Could you check a few things on this model? Use its own coordinates, in mm. A direction names the side the tool comes from. Coordinates: 2 decimals unless noted, no trailing zeros. Loops run counter-clockwise (first coordinate to the right, second up) from the corner with the lowest first, then second, coordinate; pieces in that order, holes last. Notation, with made-up numbers: M 54,-20 L 83,-20 A33 cw 83,10 Z; hole C 84,-3.75 d1. An arc over 180 degrees is marked long. Use one line per item in the form item = value. Start each with the question number.
Autodesk Inventor part; units mm, degrees
ref_plane "YZ Plane" through (0, 0, 0) normal (1, 0, 0) x (0, 1, 0)
ref_plane "XZ Plane" through (0, 0, 0) normal (0, 1, 0) x (-1, 0, 0)
ref_plane "XY Plane" through (0, 0, 0) normal (0, 0, 1) x (1, 0, 0)
sketch "Rectangle" plane through (0, 0, 0) normal (0, 1, 0) x (-1, 0, 0)
  line L0 (-48.26, -44.5) -> (48.26, -44.5)
  line L1 (48.26, -44.5) -> (48.26, 44.5)
  line L2 (48.26, 44.5) -> (-48.26, 44.5)
  line L3 (-48.26, 44.5) -> (-48.26, -44.5)
  line L4 (-48.26, -44.5) -> (48.26, 44.5) construction
  line L5 (48.26, -44.5) -> (-48.26, 44.5) construction
  point P0 (0, 0)
  dimension "d12" = 96.52
  dimension "d13" = 89
extrude "Extrusion1" add sketch "Rectangle" along normal blind 3
sketch "Sketch3" plane through (0, 3, 0) normal (0, 1, 0) x (1, 0, 0)
  line L0 (48.26, 44.5) -> (-48.26, 44.5) construction
  line L1 (-15, 44.5) -> (-5, 44.5)
  line L2 (-5, 44.5) -> (-5, 41.5)
  line L3 (-5, 41.5) -> (-15, 41.5)
  line L4 (-15, 41.5) -> (-15, 44.5)
  line L5 (0, 62.3) -> (0, -62.3) construction
  point P0 (0, 0)
  dimension "d14" = 10
  dimension "d16" = 3
  dimension "d22" = 5
extrude "Extrusion3" cut sketch "Sketch3" against normal through all
pattern_linear "Rectangular Pattern2" count 2 spacing 20 along (-1, 0, 0) count 2 spacing 40 along (1, 0, 0) of "Extrusion3"
mirror "Mirror2" about plane through (0, 0, 0) normal (0, 0, 1) of "Extrusion3", "Rectangular Pattern2"
sketch "Sketch4" plane through (0, 3, 0) normal (0, 1, 0) x (1, 0, 0)
  line L0 (67.564, 0) -> (-67.564, 0) construction
  line L1 (-48.26, 44.5) -> (-48.26, -44.5) construction
  line L2 (-48.26, 15) -> (-45.26, 15)
  line L3 (-45.26, 15) -> (-45.26, 5)
  line L4 (-45.26, 5) -> (-48.26, 5)
  line L5 (-48.26, 5) -> (-48.26, 15)
  point P0 (0, 0)
  dimension "d23" = 3
  dimension "d24" = 10
  dimension "d25" = 5
extrude "Extrusion4" cut sketch "Sketch4" against normal through all
pattern_linear "Rectangular Pattern3" count 2 spacing 20 along (0, 0, -1) count 2 spacing 40 along (0, 0, 1) of "Extrusion4"
mirror "Mirror4" about plane through (0, 0, 0) normal (1, 0, 0) of "Extrusion4", "Rectangular Pattern3"
sketch "Sketch5" plane through (0, 3, 0) normal (0, 1, 0) x (1, 0, 0)
  line L0 (48.26, 35) -> (48.26, 44.5) construction
  line L1 (48.26, 44.5) -> (35, 44.5) construction
  point P0 (0, 0)
  point P1 (36.26, 32.5)
  dimension "d31" = 12
  dimension "d32" = 12
hole "Hole1" at (36.26, 3, -32.5) direction (0, -1, 0) diameter 5 end through all
equation "\"d12\" = Module_Width"
equation "\"d13\" = Module_Height"
equation "\"d2\" = Module_Case_Thickness"
equation "\"d14\" = Module_Case_SlotWidth"
equation "\"d16\" = Module_Case_SlotDepth"
equation "\"d22\" = 0.5 * Module_Case_SlotWidth"
equation "\"d21\" = 2 * Module_Case_SlotWidth"
equation "\"d42\" = 4 * Module_Case_SlotWidth"
equation "\"d23\" = Module_Case_SlotDepth"
equation "\"d24\" = Module_Case_SlotWidth"
equation "\"d25\" = 0.5 * Module_Case_SlotWidth"
equation "\"d30\" = 2 * Module_Case_SlotWidth"
equation "\"d45\" = 4 * Module_Case_SlotWidth"
equation "\"d33\" = Module_StatusIndicatorDiameter"
equation "\"RackWidth\" = 482.6"
equation "\"U\" = 44.5"
equation "\"Module_Connector_Width\" = 6"
equation "\"Module_Case_SlotWidth\" = 10"
equation "\"Module_Case_SlotDepth\" = 3"
equation "\"Module_Back_Thickness\" = 5"
equation "\"Module_Connector_Depth\" = 4"
equation "\"Module_Height\" = 89"
equation "\"Module_Width\" = 96.52"
equation "\"Module_Case_Thickness\" = 3"
equation "\"Module_StatusIndicatorDiameter\" = 5"
equation "\"Module_Case_BottomSlotDepth\" = 5"
properties part number "BaseModule" material "Wood (Birch)"
Item 1: I want a section at B-B (z = -32.5). Write out the boundary of the cut face in (x, y).
Item 2: I want a section at D-D (x = -9.5). Write out the boundary of the cut face in (y, z).
Item 3: I want a section at C-C (z = 29.5). Write out the boundary of the cut face in (x, y), plus the area to 3 significant figures.
Item 4: Thinking about a two-plate mould opening in X: for faces 6 (the flat face through (-10, 2, -41.5)), 7 (the flat face through (48.26, 1, 0)), 8 (the flat face through (20, 1, -44.5)), which applies, pulls with the +X half, pulls with the -X half, needs draft (parallel to the pull), parting line crosses it, or undercut?
Item 5: For faces 1 (the flat face through (25, 2, 43)), 2 (the flat face through (-45.26, 2, -30)), 3 (the flat face through (1, 3, 1)), 4 (the flat face through (25, 2, -43)), 5 (the flat face through (47, 2, 35)), which set-ups out of +Z, -Z, +X, -X, +Y, -Y let a thin tool reach every point of the face, with its end or its side?
Item 6: I want a section at A-A (x = 36.26). Write out the boundary of the cut face in (y, z), plus the area to 3 significant figures.
Item 7: Please list where these lines run through material, in increasing order: line 1 along Z through (x, y) = (36.26, 1.75); line 2 along X through (y, z) = (1.5, -32.5); line 3 along X through (y, z) = (1, 10.5).
Item 8: I'm going to push flat-ended pins straight in: P1, Ø1.5, axis at y = 2, z = -11, coming from the -X side; P2, Ø0.9, axis at x = -30.5, y = 1.5, coming from the -Z side; P3, Ø0.9, axis at x = 29.5, y = 1.5, coming from the +Z side. Where does each tip first touch, or does it pass through?
Worked answers:
q1.outline = M -45.26,0 L 33.76,0 L 33.76,3 L -45.26,3 Z; M 38.76,0 L 45.26,0 L 45.26,3 L 38.76,3 Z
q2.outline = M 0,-41.5 L 3,-41.5 L 3,41.5 L 0,41.5 Z
q3.outline = M -45.26,0 L 45.26,0 L 45.26,3 L -45.26,3 Z
q3.area = 272 mm²
q4.face_6 = undercut
q4.face_7 = pulls with the +X half
q4.face_8 = needs draft
q5.face_1 = +Z, +Y, -Y
q5.face_2 = -X, +Y, -Y
q5.face_3 = +Z, -Z, +X, -X, +Y
q5.face_4 = -Z, +Y, -Y
q5.face_5 = +X, +Y, -Y
q6.outline = M 0,-44.5 L 3,-44.5 L 3,-35 L 0,-35 Z; M 0,-30 L 3,-30 L 3,44.5 L 0,44.5 Z
q6.area = 252 mm²
q7.line_1 = -44.5 to -35, -30 to 44.5
q7.line_2 = -45.26 to 33.76, 38.76 to 45.26
q7.line_3 = -45.26 to 45.26
q8.P1 = -45.26
q8.P2 = -41.5
q8.P3 = 41.5
